```python
from build123d import *

# Parameters (mm, degrees)
SKETCH1_R           = 6.861165386
SKETCH1_R_2         = 18.200911839
SKETCH1_R_3         = 11.1125
SKETCH1_R_4         = 2.5527
BOSS_EXTRUDE1_DEPTH = 5.55625
FILLET1_R           = 25.4
FILLET3_R           = 12.7
FILLET4_R           = 12.7


with BuildPart() as part:
    # Sketch1 → Boss-Extrude1 (new body)
    with BuildSketch(Plane.XY):
        with BuildLine():
            Line((198.861588808, 69.615973931), (188.964925061, 57.285610842))
            Line((188.964925061, 57.285610842), (205.711419625, 50.270822653))
            Line((205.711419625, 50.270822653), (208.580766503, 42.167272229))
            Line((208.580766503, 42.167272229), (200.684125291, -98.616772294))
            Line((200.684125291, -98.616772294), (189.611167808, -151.385643895))
            Line((189.611167808, -151.385643895), (38.107034572, -236.120024372))
            ThreePointArc((38.107034572, -236.120024372), (1.581834572, -199.594824372), (38.107034572, -163.069624372))
            Line((38.107034572, -163.069624372), (103.581383992, -139.886129452))
            Line((103.581383992, -139.886129452), (147.550432491, -89.7457244))
            Line((147.550432491, -89.7457244), (171.836242771, -16.814689905))
            Line((171.836242771, -16.814689905), (178.189444477, 2.26417003))
            Line((178.189444477, 2.26417003), (167.830043749, 27.447208055))
            Line((167.830043749, 27.447208055), (157.470643022, 73.010133983))
            Line((157.470643022, 73.010133983), (157.470643022, 93.390021886))
            Line((157.470643022, 93.390021886), (170.600142232, 98.791028052))
            Line((170.600142232, 98.791028052), (190.927975242, 92.021922153))
            Line((190.927975242, 92.021922153), (198.861588808, 69.615973931))
        make_face()
        with Locations((38.107034572, -199.594824372)):
            Circle(SKETCH1_R, mode=Mode.SUBTRACT)
        with Locations((161.686314612, -124.719021489)):
            Circle(SKETCH1_R_2, mode=Mode.SUBTRACT)
        with Locations((188.964925061, 29.396113336)):
            Circle(SKETCH1_R_3, mode=Mode.SUBTRACT)
        with Locations((173.035965272, 78.237579188)):
            Circle(SKETCH1_R_3, mode=Mode.SUBTRACT)
        with Locations((38.107034572, -174.194824372)):
            Circle(SKETCH1_R_4, mode=Mode.SUBTRACT)
        with Locations((63.507034572, -199.594824372)):
            Circle(SKETCH1_R_4, mode=Mode.SUBTRACT)
        with Locations((38.107034572, -224.994824372)):
            Circle(SKETCH1_R_4, mode=Mode.SUBTRACT)
        with Locations((12.707034572, -199.594824372)):
            Circle(SKETCH1_R_4, mode=Mode.SUBTRACT)
    extrude(amount=BOSS_EXTRUDE1_DEPTH)

    # Fillet1
    # the kernel refuses this fillet: 25.4 mm, written as the material it adds along each edge
    with BuildSketch(Plane(origin=(178.189444477, 2.26417003, 0), x_dir=(-0.38043310119112933, 0.9248084426074947, 0), z_dir=(0, 0, 1))) as fillet1_piece_1:
        with BuildLine():
            CenterArc((FILLET1_R * 0.371679258358, FILLET1_R), FILLET1_R, 229.221887669, 40.778112331)
            Line((-FILLET1_R * 0.281452116845, FILLET1_R * 0.242755385146), (0, 0))
            Line((0, 0), (FILLET1_R * 0.371679258358, 0))
        make_face()
    extrude(amount=5.55625)
    with BuildSketch(Plane(origin=(147.550432491, -89.7457244, 0), x_dir=(0.315940492730092, 0.948779007489872, 0), z_dir=(0, 0, 1))) as fillet1_piece_2:
        with BuildLine():
            CenterArc((FILLET1_R * 0.201912574353, FILLET1_R), FILLET1_R, 247.169477311, 22.830522689)
            Line((-FILLET1_R * 0.186094053331, FILLET1_R * 0.0783434170618), (0, 0))
            Line((0, 0), (FILLET1_R * 0.201912574353, 0))
        make_face()
    extrude(amount=5.55625)
    with BuildSketch(Plane(origin=(103.581383992, -139.886129452, 0), x_dir=(-0.9426514039125685, -0.333778864971501, 0), z_dir=(0, 0, 1))) as fillet1_piece_3:
        with BuildLine():
            CenterArc((FILLET1_R * 0.26097983986, -FILLET1_R), FILLET1_R, 90, 29.253579042)
            Line((-FILLET1_R * 0.22769590207, -FILLET1_R * 0.127534516872), (0, 0))
            Line((0, 0), (FILLET1_R * 0.26097983986, 0))
        make_face()
    extrude(amount=5.55625)
    with BuildSketch(Plane(origin=(38.107034572, -163.069624372, 0), x_dir=(0.9426514039125696, 0.3337788649714982, 0), z_dir=(0, 0, 1))) as fillet1_piece_4:
        with BuildLine():
            CenterArc((3.778567788, 25.4), FILLET1_R, 255.05508403, 14.94491597)
            ThreePointArc((-2.771845496, 0.85917512), (-1.377386631, 0.457126529), (0, 0))
            Line((0, 0), (3.778567788, 0))
        make_face()
    extrude(amount=5.55625)
    # the kernel refuses this fillet: 25.4 mm, written as the material it takes off along each edge
    with BuildSketch(Plane(origin=(157.470643022, 93.390021886, -42.096203676), x_dir=(0, -1, 0), z_dir=(0, 0, 1))) as fillet1_2_piece_1:
        with BuildLine():
            CenterArc((16.83848147, 25.4), FILLET1_R, 208.887448124, 61.112551876)
            Line((-5.401006167, 13.12949921), (0, 0))
            Line((0, 0), (16.83848147, 0))
        make_face()
    extrude(amount=89.748657352, mode=Mode.SUBTRACT)
    with BuildSketch(Plane(origin=(157.470643022, 73.010133983, -7.12787144), x_dir=(0.22170637645104777, -0.9751134716744232, 0), z_dir=(0, 0, 1))) as fillet1_2_piece_2:
        with BuildLine():
            CenterArc((FILLET1_R * 0.11224994393, FILLET1_R), FILLET1_R, 257.190723516, 12.809276484)
            Line((-FILLET1_R * 0.109456432521, FILLET1_R * 0.0248865283256), (0, 0))
            Line((0, 0), (FILLET1_R * 0.11224994393, 0))
        make_face()
    extrude(amount=19.811992879, mode=Mode.SUBTRACT)
    with BuildSketch(Plane(origin=(167.830043749, 27.447208055, -5.305032246), x_dir=(0.3804331011911332, -0.9248084426074932, 0), z_dir=(0, 0, 1))) as fillet1_2_piece_3:
        with BuildLine():
            CenterArc((FILLET1_R * 0.0835438149047, FILLET1_R), FILLET1_R, 260.448763965, 9.551236035)
            Line((-FILLET1_R * 0.0823856984158, FILLET1_R * 0.0138623845481), (0, 0))
            Line((0, 0), (FILLET1_R * 0.0835438149047, 0))
        make_face()
    extrude(amount=16.166314493, mode=Mode.SUBTRACT)
    with BuildSketch(Plane(origin=(38.107034572, -236.120024372, -39.792317969), x_dir=(0.8727709569033328, 0.48812995891057614, 0), z_dir=(0, 0, 1))) as fillet1_2_piece_4:
        with BuildLine():
            CenterArc((8.784495846, 25.4), FILLET1_R, 215.61203078, 54.38796922)
            ThreePointArc((-11.865158329, 10.609740285), (-6.517544718, 4.650687408), (0, 0))
            Line((0, 0), (8.784495846, 0))
        make_face()
    extrude(amount=85.140885938, mode=Mode.SUBTRACT)
    with BuildSketch(Plane(origin=(189.611167808, -151.385643895, -28.892669195), x_dir=(0.20536614533433253, 0.9786852131050707, 0), z_dir=(0, 0, 1))) as fillet1_2_piece_5:
        with BuildLine():
            CenterArc((FILLET1_R * 0.455002664481, FILLET1_R), FILLET1_R, 221.068676821, 48.931323179)
            Line((-FILLET1_R * 0.298919997384, FILLET1_R * 0.343036819962), (0, 0))
            Line((0, 0), (FILLET1_R * 0.455002664481, 0))
        make_face()
    extrude(amount=63.341588389, mode=Mode.SUBTRACT)
    with BuildSketch(Plane(origin=(200.684125291, -98.616772294, -4.797187782), x_dir=(0.056002429151398234, 0.9984306325074078, 0), z_dir=(0, 0, 1))) as fillet1_2_piece_6:
        with BuildLine():
            CenterArc((FILLET1_R * 0.075546264279, FILLET1_R), FILLET1_R, 261.359448749, 8.640551251)
            Line((-FILLET1_R * 0.0746888367943, FILLET1_R * 0.0113497006497), (0, 0))
            Line((0, 0), (FILLET1_R * 0.075546264279, 0))
        make_face()
    extrude(amount=15.150625563, mode=Mode.SUBTRACT)
    with BuildSketch(Plane(origin=(208.580766503, 42.167272229, -12.751193258), x_dir=(-0.33377886497150366, 0.9426514039125676, 0), z_dir=(0, 0, 1))) as fillet1_2_piece_7:
        with BuildLine():
            CenterArc((FILLET1_R * 0.200806193046, FILLET1_R), FILLET1_R, 247.291319111, 22.708680889)
            Line((-FILLET1_R * 0.185239618687, FILLET1_R * 0.0775203897954), (0, 0))
            Line((0, 0), (FILLET1_R * 0.200806193046, 0))
        make_face()
    extrude(amount=31.058636517, mode=Mode.SUBTRACT)

    # Fillet3
    fillet3_edges = [part.edges().sort_by_distance(p)[0] for p in [
        (170.600142232, 98.791028052, 2.778125),
        (190.927975242, 92.021922153, 2.778125),
    ]]
    fillet(fillet3_edges, radius=FILLET3_R)

    # Fillet4
    fillet4_edges = [part.edges().sort_by_distance(p)[0] for p in [
        (205.711419625, 50.270822653, 2.778125),
        (198.861588808, 69.615973931, 2.778125),
    ]]
    fillet(fillet4_edges, radius=FILLET4_R)


solid = part.part
```
Input: part model. Units: mm. Frame: model coordinates. A direction names the side the tool comes from. Give positions to 0.01 mm unless a question says otherwise; leave off trailing zeros. Order: outer loops, then holes, each group sorted by start corner. A loop starts at its lowest first (then second) coordinate and runs counter-clockwise, first axis right, second up. Notation, with made-up numbers: M 77.25,30.25 L 84.25,30.25 A5 cw 84.25,35.25 Z; hole C -38,67.5 d9. An arc over 180 degrees is marked long. One line per question, with ' | ' between items. Start each with the question number.
1. First-contact query: pin 1 Ø2 at (y, z) = (-54, 1) entering from +X; pin 2 Ø1 at (x, z) = (86, 2) entering from -Y; pin 3 Ø0.8 at (y, z) = (76, 3) entering from -X. Flat tips, straight axial feed; report the tip coordinate or a pass-through.
2. Pull-direction query (X, two-part tool) for faces 1 (the face through (204.596, -28.877, 2.739)), 2 (the face through (162.796, 49.588, 2.739)), 3 (the face through (41.273, -205.682, 2.739)); classes: released by +X, released by -X, zero draft, split by the parting line, or undercut.
3. Material intervals for probe 1 along Y at (x, z) = (39, 3.7); probe 2 along X at (y, z) = (30.5, 2.7); probe 3 along Y at (x, z) = (145, 3.5), sorted ascending. Write a range as [from, to].
4. Section query A-A (z = 2.6). Count the separate pieces of the cut face and the enclosed holes in it, and give its area (3 significant figures).
5. Section query C-C (x = 115). Return the cut outline in (y, z), and give its area (3 significant figures).
6. Access query for faces 4 (the face through (69.11, -152.09, 2.74)), 5 (the face through (171.66, 18.14, 2.74)). Directions: +Z, -Z, +X, -X, +Y, -Y. A direction counts if a zero-diameter tool reaches every point of the face in a straight line with its end or side. Return the directions, or none.
7. Section query B-B (y = -76.5). Return the cut outline in (x, z).
Here are the results:
1) pin 1: x = 203.24 | pin 2: y = -209.61 | pin 3: x = 157.47
2) face 1: released by +X | face 2: released by -X | face 3: undercut
3) probe 1: [-234.43, -227.39], [-222.6, -206.4], [-192.79, -176.59], [-171.8, -162.59] | probe 2: [167.14, 177.91], [200.02, 207.93] | probe 3: [-176.34, -131.99], [-117.45, -92.6]
4) separate pieces: 1 | enclosed holes: 8 | area: 18,200 mm²
5) outline: M -193.11,0 L -126.86,0 L -126.86,5.56 L -193.11,5.56 Z | area: 368 mm²
6) face 4: +Z, -Z, -X, +Y | face 5: +Z, -Z, -X
7) outline: M 151.96,0 L 201.92,0 L 201.92,5.56 L 151.96,5.56 Z
